Work out the finished part from the listing and answer in its coordinate system (mm). A direction names the side the tool comes from. Coordinates: 2 decimals unless noted, no trailing zeros. Order: outer loops, then holes, each group sorted by start corner. A loop starts at its lowest first (then second) coordinate and runs counter-clockwise, first axis right, second up. Notation, with made-up numbers: (84, 8.25) - (96, 8.25) arc R22 cw to (96, 46.25) - close; hole circle Ø4 at (-29, -2). An arc over 180 degrees is marked (long way). Use CSV: the item, a comma, the result in double quotes. Start each with the question number.
Autodesk Inventor part; units mm, degrees
ref_plane "YZ Plane" through (0, 0, 0) normal (1, 0, 0) x (0, 1, 0)
ref_plane "XZ Plane" through (0, 0, 0) normal (0, 1, 0) x (-1, 0, 0)
ref_plane "XY Plane" through (0, 0, 0) normal (0, 0, 1) x (1, 0, 0)
sketch "Skizze1" plane through (0, 0, 0) normal (0, 1, 0) x (-1, 0, 0)
  circle A0 centre (11.4284, -11.664) radius 5
  circle A1 centre (11.4284, -11.664) radius 2.5
  point P0 (0, 0)
  dimension "d0" = 10
  dimension "d1" = 5
extrude "Extrusion1" add sketch "Skizze1" along normal blind 150 contours A0 | A1
extrude "Extrusion2" add sketch "Skizze1" against normal blind 3 contours A1
thread "Gewinde1"
sketch "Skizze2" plane through (-11.4284, 150, -11.664) normal (0, 1, 0) x (1, 0, 0)
  point P0 (11.4284, -11.664)
  point P1 (0, 0)
hole "Bohrung1" at (-11.4284, 150, -11.664) direction (0, -1, 0) diameter 4.978 depth 19.05 tip angle 118
properties part number "Stangen"
1) For a pull along Z with two mould halves and no side action, classify faces 1 (the face through (-10.886, -1.479, -14.105)), 2 (the face through (-9, 150, -13)), 3 (the face through (-11.299, 129.714, -11.252)) as +Z half, -Z half, draft (parallel to the pull), parting line (faces both ways), or undercut.
2) For faces 4 (the face through (-11, -3, -12)), 5 (the face through (-13.896, 140.342, -11.988)), 6 (the face through (-9, 0, -13)), determine the directions among +Z, -Z, +X, -X, +Y, -Y from which every point of the face is accessible in a straight line to the end or side of a thin tool.
3) Straight lines are drawn through the part: line 1 (Y direction, x = -7.75, z = -9.5); line 2 (X direction, y = 18.5, z = -11.5); line 3 (Z direction, x = -13.75, y = 80.5). For each, find the intervals that lie inside material, in ascending order. Write a range as [from, to].
4) The part is cut by section A-A on y = 119.5. Determine the outline of the cut face in (x, z), plus the area to 3 significant figures.
5) Flat-ended cylindrical pins translate along their axes: P1, Ø2, axis at x = -9, y = 91.5, coming from the -Z side; P2, Ø1.5, axis at x = -7.5, y = 73.5, coming from the -Z side. Find the tip coordinate at first contact, or state that the pin passes through.
Answer key:
1,face 1,"parting line"
1,face 2,"draft"
1,face 3,"undercut"
2,face 4,"+Z, -Z, +X, -X, -Y"
2,face 5,"+Y"
2,face 6,"-Y"
3,line 1,"[0, 150]"
3,line 2,"[-16.43, -6.43]"
3,line 3,"[-16.09, -7.24]"
4,outline,"circle Ø10 at (-11.43, -11.66)"
4,area,"78.5 mm^2"
5,P1,"z = -16.46"
5,P2,"z = -15.52"
